Part model, mm, in its own coordinate system. A direction names the side the tool comes from. Coordinates: 2 decimals unless noted, no trailing zeros. Write each loop counter-clockwise with the first axis right and the second up, starting at its lowest first coordinate (ties: lowest second). Pieces come first, ordered by that corner, then holes. Notation, with made-up numbers: (-28.5, 54) -> (-8.5, 54) arc R29 ccw to (-8.5, 82) -> close; hole circle Ø6 at (-4.75, -3). An arc over 180 degrees is marked (long way). Write item = value, one per line.
from build123d import *

# Parameters (mm, degrees)
SKETCH1_R           = 1.5875
SKETCH1_R_2         = 3
SKETCH1_R_3         = 3.2385
SKETCH1_W           = 33.02
SKETCH1_H           = 4.7625
BOSS_EXTRUDE1_DEPTH = 4.7625
CHAMFER1_SIZE       = 5.08


with BuildPart() as part:
    # Sketch1 → Boss-Extrude1 (new body)
    with BuildSketch(Plane(origin=(0, 0, 0), x_dir=(0, 0, -1), z_dir=(1, 0, 0))):
        Polygon((-58.293, 118.7905), (58.293, 118.7905), (58.293, 110.6625), (50.293, 110.6625), (50.293, 105.9), (58.293, 105.9), (58.293, 72.5625), (50.293, 72.5625), (50.293, 67.8), (58.293, 67.8), (58.293, 42.8625), (50.293, 42.8625), (50.293, 38.1), (58.293, 38.1), (58.293, -38.1), (50.293, -38.1), (50.293, -42.8625), (58.293, -42.8625), (58.293, -66.374), (38.857, -66.374), (38.857, -97.87), (58.293, -97.87), (58.293, -105.9), (50.293, -105.9), (50.293, -110.6625), (58.293, -110.6625), (58.293, -118.7905), (-58.293, -118.7905), (-58.293, -110.6625), (-50.293, -110.6625), (-50.293, -105.9), (-58.293, -105.9), (-58.293, -72.5625), (-50.293, -72.5625), (-50.293, -67.8), (-58.293, -67.8), (-58.293, -42.8625), (-50.293, -42.8625), (-50.293, -38.1), (-58.293, -38.1), (-58.293, 38.1), (-50.293, 38.1), (-50.293, 42.8625), (-58.293, 42.8625), (-58.293, 67.8), (-50.293, 67.8), (-50.293, 72.5625), (-58.293, 72.5625), (-58.293, 105.9), (-50.293, 105.9), (-50.293, 110.6625), (-58.293, 110.6625), align=None)
        with Locations((3, 9.519071488)):
            Circle(SKETCH1_R, mode=Mode.SUBTRACT)
        with Locations((-6.519071488, 0)):
            Circle(SKETCH1_R, mode=Mode.SUBTRACT)
        with Locations((3, -9.519071488)):
            Circle(SKETCH1_R, mode=Mode.SUBTRACT)
        with Locations((3, 0)):
            Circle(SKETCH1_R_2, mode=Mode.SUBTRACT)
        with Locations((-35.174, -17.15)):
            Circle(SKETCH1_R_3, mode=Mode.SUBTRACT)
        with Locations((-49.398, -17.15)):
            Circle(SKETCH1_R_3, mode=Mode.SUBTRACT)
        with Locations((-45.464, -58.872973782)):
            Circle(SKETCH1_R_3, mode=Mode.SUBTRACT)
        with Locations((0, 108.28125)):
            Rectangle(SKETCH1_W, SKETCH1_H, mode=Mode.SUBTRACT)
        with Locations((0, 70.18125)):
            Rectangle(SKETCH1_W, SKETCH1_H, mode=Mode.SUBTRACT)
        with Locations((0, 40.48125)):
            Rectangle(SKETCH1_W, SKETCH1_H, mode=Mode.SUBTRACT)
        with Locations((0, -40.48125)):
            Rectangle(SKETCH1_W, SKETCH1_H, mode=Mode.SUBTRACT)
        with Locations((0, -70.18125)):
            Rectangle(SKETCH1_W, SKETCH1_H, mode=Mode.SUBTRACT)
        with Locations((0, -108.28125)):
            Rectangle(SKETCH1_W, SKETCH1_H, mode=Mode.SUBTRACT)
    extrude(amount=-BOSS_EXTRUDE1_DEPTH)

    # Chamfer1
    chamfer1_edges = [part.edges().sort_by_distance(p)[0] for p in [
        (-2.38125, 118.7905, 58.293),
        (-2.38125, 118.7905, -58.293),
        (-2.38125, -118.7905, -58.293),
        (-2.38125, -118.7905, 58.293),
    ]]
    chamfer(chamfer1_edges, length=CHAMFER1_SIZE)


solid = part.part
Q1. Saw through at C-C on x = -2.7. Count the separate pieces of the cut face and the enclosed holes in it, and give its area (3 significant figures).
Model answer:
separate_pieces = 1
enclosed_holes = 13
area = 25,500 mm²
Q2. Saw through at A-A on y = -17.15. Give the cut face in (x, z), and give its area (3 significant figures).
Model answer:
outline = (-4.76, -58.29) -> (0, -58.29) -> (0, 31.94) -> (-4.76, 31.94) -> close; (-4.76, 38.41) -> (0, 38.41) -> (0, 46.16) -> (-4.76, 46.16) -> close; (-4.76, 52.64) -> (0, 52.64) -> (0, 58.29) -> (-4.76, 58.29) -> close
area = 494 mm²
Q3. Mould opens along Z. For faces 1 (the face through (-2, -56, 58.293)), 2 (the face through (-2, -67.8, 0)), 3 (the face through (-2, 110.662, 54)) say: released by +Z, released by -Z, zero draft, split by the parting line, or undercut.
Model answer:
face_1 = released by +Z
face_2 = undercut
face_3 = zero draft
Q4. Pin check, flat tips, straight feed: pin 1 (1.4 mm diameter, centred on x = -3.5, y = 107, fed in from +Z); pin 2 (2.5 mm diameter, centred on x = -1.5, y = -71, fed in from -Z); pin 3 (1.4 mm diameter, centred on x = -2.5, y = 69.5, fed in from -Z). Stop position of each tip, or through.
Model answer:
pin_1 = 50.29
pin_2 = -38.86
pin_3 = -50.29
Q5. Saw through at B-B on z = -41.5. Give the cut face in (x, y).
Model answer:
outline = (-4.76, -118.79) -> (0, -118.79) -> (0, -97.87) -> (-4.76, -97.87) -> close; (-4.76, -66.37) -> (0, -66.37) -> (0, 118.79) -> (-4.76, 118.79) -> close
Q6. Probe line 1 (Z direction, x = -3.5, y = -42.5); line 2 (Y direction, x = -1.75, z = 42.5); line 3 (Y direction, x = -3.15, z = 36). List the from-to ranges inside material, lowest first. Write a range as from..to.
Model answer:
line_1 = -50.29..-16.51, 16.51..50.29
line_2 = -118.79..-60.18, -57.57..118.79
line_3 = -118.79..-20.28, -14.02..118.79
Q7. Which spindle directions (+Z, -Z, +X, -X, +Y, -Y) get a long thin tool onto all of the face, cutting with end or side? Do faces 4 (the face through (-2, -40, -50.293)), 5 (the face through (-2, 42.862, 54)), 6 (the face through (-2, -118.79, -1)), 7 (the face through (-2, 55, 58.293)), 8 (the face through (-2, -41, -16.51)). Say none if no direction does.
Model answer:
face_4 = -Z, +X, -X
face_5 = +Z, +X, -X
face_6 = +Z, -Z, +X, -X, -Y
face_7 = +Z, +X, -X, +Y, -Y
face_8 = +X, -X
